from build123d import *

# Parameters (mm, degrees)
F0_R     = 11.2
F1_DEPTH = 7
F2_R     = 1.5


with BuildPart() as f1:
    # F0 (on Top) → F1 (new body)
    with BuildSketch(Plane.XY):
        with BuildLine():
            Line((-13.1840748528, 25.7517945722), (-13.1840748528, 0.6482054278))
            Line((-13.1840748528, 0.6482054278), (-13.1840748528, -0.6482054278))
            Line((-13.1840748528, -0.6482054278), (-13.1840748528, -26.2634836304))
            Line((-13.1840748528, -26.2634836304), (-13.1840748528, -26.5365075959))
            ThreePointArc((-13.1840748528, -26.5365075959), (0.0853785885, -39.5998091598), (13.215218689, -26.3961906666))
            Line((13.215218689, -26.3961906666), (13.2, 26.4))
            ThreePointArc((13.2, 26.4), (0.3242005116, 39.5960181126), (-13.1840748528, 27.0482054278))
            Line((-13.1840748528, 27.0482054278), (-13.1840748528, 25.7517945722))
        make_face()
        Circle(F0_R, mode=Mode.SUBTRACT)
        with Locations((0.0152192374, -26.3999956132)):
            Circle(F0_R, mode=Mode.SUBTRACT)
        with Locations((0, 26.4)):
            Circle(F0_R, mode=Mode.SUBTRACT)
    extrude(amount=F1_DEPTH)

    # F2
    f2_edges = [f1.edges().sort_by_distance(p)[0] for p in [
        (0.085379, -39.599809, 0),
        (0.324201, 39.596018, 0),
        (0.324201, 39.596018, 7),
        (-13.184075, 0.255849, 7),
        (13.207609, 0.001905, 7),
        (13.207609, 0.001905, 0),
        (-13.184075, 0.255849, 0),
        (0.085379, -39.599809, 7),
    ]]
    fillet(f2_edges, radius=F2_R)


solid = f1.part
Can you work these out from the model? Positions are in its coordinate system, mm. Give positions to 0.01 mm unless a question says otherwise; leave off trailing zeros. Order: outer loops, then holes, each group sorted by start corner. A loop starts at its lowest first (then second) coordinate and runs counter-clockwise, first axis right, second up. Notation, with made-up numbers: M 51.5,-15.75 L 58.5,-15.75 A25 ccw 58.5,4.25 Z; hole C 57,49 d4. An arc over 180 degrees is marked long. Use one line per item in the form item = value.
Item 1: If we section it at B-B, the plane x = -6: Count the separate pieces of the cut face and the enclosed holes in it, and give its area (3 significant figures).
Values follow:
separate_pieces = 4
enclosed_holes = 0
area = 135 mm^2
Item 2: Will these pins go through, and if not, where does the flat tip stop? pin 1 Ø3 at (x, z) = (3, 3) entering from -Y; pin 2 Ø1.2 at (y, z) = (9.5, 3) entering from +X.
Values follow:
pin_1 = -39.52
pin_2 = 13.21
Item 3: If we section it at A-A, the plane z = 4.75: Write out the boundary of the cut face in (x, y), and give its area (3 significant figures).
Values follow:
outline = M -13.18,-26.54 A13.2 ccw 13.22,-26.4 L 13.2,26.4 A13.2 ccw -13.18,27.05 Z; hole C 0,0 d22.4; hole C 0,26.4 d22.4; hole C 0.02,-26.4 d22.4
area = 759 mm^2
Item 4: Thinking about a two-plate mould opening in Y: for faces 1 (the cylindrical face through (12.78, 0.37, 6.55)), 2 (the flat face through (0.8, 11.5, 0)), 3 (the cylindrical face through (-11.19, 0.49, 3.45)), which applies, pulls with the +Y half, pulls with the -Y half, needs draft (parallel to the pull), parting line crosses it, or undercut?
Values follow:
face_1 = pulls with the +Y half
face_2 = needs draft
face_3 = undercut
Item 5: If I drill on line 1 along Y through (x, z) = (5, 2.5); line 2 along Y through (x, z) = (0, 3); line 3 along X through (y, z) = (27, 3), over which ranges is the centre line in solid material (lowest first)? Write a range as [from, to].
Values follow:
line_1 = [-38.62, -36.43], [-16.37, -10.02], [10.02, 16.38], [36.42, 38.62]
line_2 = [-39.6, -37.6], [-15.2, -11.2], [11.2, 15.2], [37.6, 39.6]
line_3 = [-13.18, -11.18], [11.18, 13.19]
